Here's the drawing with two shaded views (mm, measured from the low corner). I have some questions. Give positions to 0.01 mm unless a question says otherwise; leave off trailing zeros. Loops run counter-clockwise (first coordinate to the right, second up) from the corner with the lowest first, then second, coordinate; pieces in that order, holes last. Notation, with made-up numbers: M -1,22.5 L 34,22.5 A19 ccw 34,48.5 Z; hole C 18,44 d7. An arc over 180 degrees is marked long. Use CSV: the item, a comma, the result in double quotes.
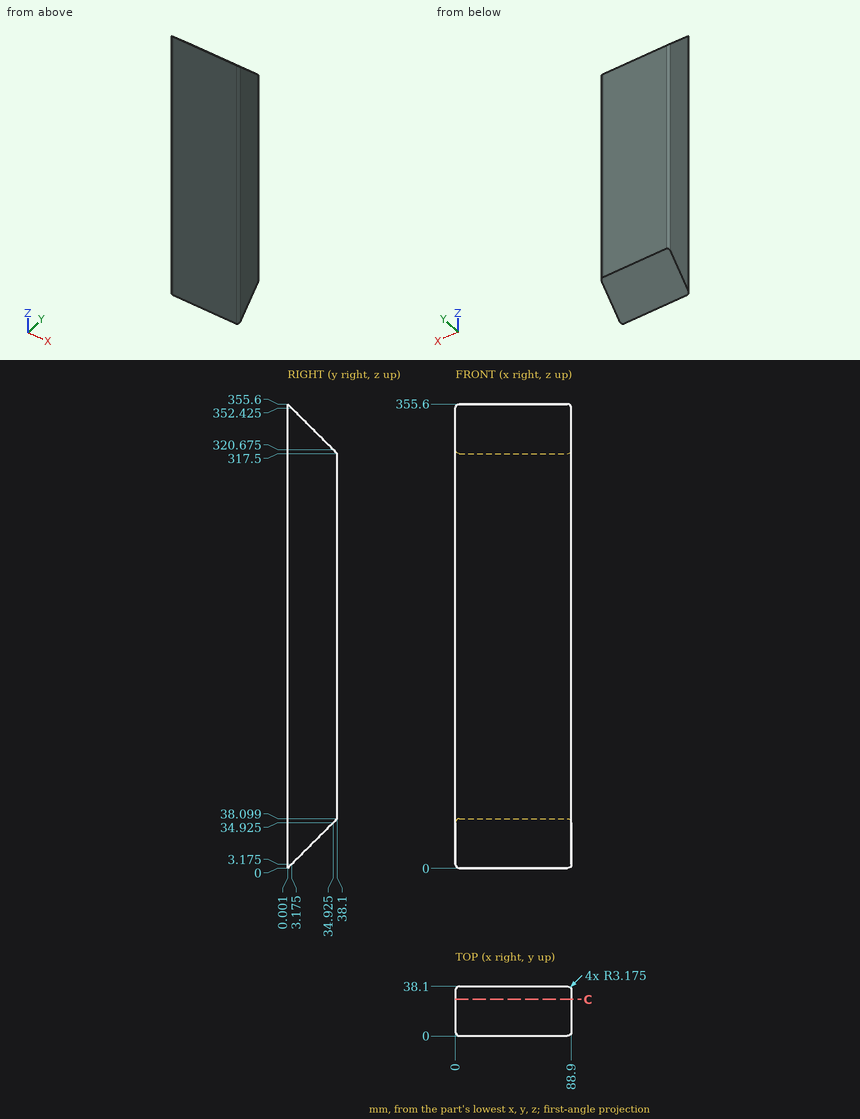
1. I'm going to push flat-ended pins straight in: pin 1 Ø4 at (x, y) = (19.5, 4) entering from +Z; pin 2 Ø2 at (x, y) = (23.5, 10) entering from +Z; pin 3 Ø10 at (x, y) = (72.5, 13) entering from +Z. Where does each tip first touch, or does it pass through?
Outcome:
pin 1,"z = 353.6"
pin 2,"z = 346.6"
pin 3,"z = 347.6"
2. I want a section at C-C, the plane y = 28. List the corners of the cut face in (x, z) for me.
Outcome:
outline,"M 0,28 L 88.9,28 L 88.9,327.6 L 0,327.6 Z"
3. Please list where these lines run through material, in increasing order: line 1 (X direction, y = 3, z = 57.5) (1 decimal); line 2 (Z direction, x = 59, y = 34); line 3 (Z direction, x = 43, y = 21).
Outcome:
line 1,"0 to 88.9"
line 2,"34 to 321.6"
line 3,"21 to 334.6"
